Input: part model. Units: mm. Frame: model coordinates. A direction names the side the tool comes from. Round coordinates to 2 decimals unless told otherwise and drop trailing zeros. Loops run counter-clockwise (first coordinate to the right, second up) from the corner with the lowest first, then second, coordinate; pieces in that order, holes last. Notation, with made-up numbers: M 32.5,-39.5 L 39.5,-39.5 A33 cw 39.5,-0.5 Z; hole C 78,57 d3. An arc over 180 degrees is marked long. Return JSON: item names as keys, results as strings. Group by question number.
1) Material intervals for line 1 (Y direction, x = 4, z = 0.5); line 2 (Z direction, x = -3.5, y = 0); line 3 (Y direction, x = 1, z = 2.75), sorted ascending. Write a range as from..to.
2) Section B-B (z = -1.5). Output: boundary loops of the cut face in (x, y), plus the area to 3 significant figures.
3) Contact query for flat-ended pins moving along their axis: P1, Ø1.5, axis at y = -0.5, z = 0.5, coming from the +X side; P2, Ø3.5, axis at x = 0.5, y = 3, coming from the -Z side; P3, Ø0.7, axis at y = -6.5, z = 1, coming from the -X side. Output: stop coordinate, or through.
4) Section C-C (y = 2.75). Output: boundary loops of the cut face in (x, z).
5) Section A-A (x = -11). Output: boundary loops of the cut face in (y, z).
6) Mould query, pull axis X, two halves, no side actions, for faces 1 (the face through (-16.68, -0.02, 0.59)), 2 (the face through (6, -5.817, 1)), 3 (the face through (0, 0, 0)). Classes: +X half, -X half, draft (parallel to the pull), parting line (faces both ways), or undercut.
7) Access query for faces 4 (the face through (0, 0, 1.2)), 5 (the face through (-17.164, -5.753, 0.592)), 6 (the face through (13.42, 1.36, 0.59)). Directions: +Z, -Z, +X, -X, +Y, -Y. A direction counts if a zero-diameter tool reaches every point of the face in a straight line with its end or side. Return the directions, or none.
from build123d import *

# Parameters (mm, degrees)
EXTRUDE_1_DEPTH     = 1.2
CUT_EXTRUDE_START   = -1.2
CUT_EXTRUDE_1_DEPTH = 1.2
SKETCH_3_R          = 0.6
EXTRUDE_2_DEPTH     = 0.3
SKETCH_4_W          = 31.58406245
SKETCH_4_H          = 7.800680058
EXTRUDE_3_DEPTH     = 0.6


# Read off the part's stored shape, not the designer's step: Вырез-Вытянуть-Тонкостенный1
with BuildPart() as part:
    # Эскиз1 → Бобышка-Вытянуть1 (new body)
    with BuildSketch(Plane.XY):
        with BuildLine():
            Line((-18.4888994, -6.081212357), (-16.002013835, -6.217213911))
            Line((-16.002013835, -6.217213911), (10.732005982, -6.217213911))
            add(Edge.make_bspline(
                [(10.732005982, -6.217213911), (11.47341135, -6.18385268), (12.922426791, -6.118650915), (15.00936311, -5.600631561), (16.935457079, -4.747576966), (18.044624718, -3.914711141), (18.600667338, -3.497182825)],
                knots=[0, 0, 0, 0, 0.261630689, 0.511335532, 0.755025064, 1, 1, 1, 1], degree=3))
            Line((18.600667338, -3.497182825), (18.870975113, -3.202301616))
            Line((18.870975113, -3.202301616), (8.829771562, 6.217213911))
            Line((8.829771562, 6.217213911), (-15.234306629, 6.217213911))
            Line((-15.234306629, 6.217213911), (-18.870975113, -5.962739267))
            Line((-18.870975113, -5.962739267), (-18.4888994, -6.081212357))
        make_face()
    extrude(amount=EXTRUDE_1_DEPTH)

    # Вырез-Вытянуть-Тонкостенный1 outline → Вырез-Вытянуть-Тонкостенный1 (cut)
    with BuildSketch(Plane.XY.offset(1.2).offset(CUT_EXTRUDE_START)):
        with BuildLine():
            Line((-16.002013835, -6.217213911), (10.732005982, -6.217213911))
            add(Edge.make_bspline(
                [(10.732005982, -6.217213911), (11.47341135, -6.18385268), (12.922426791, -6.118650915), (15.00936311, -5.600631561), (16.935457079, -4.747576966), (18.044624718, -3.914711141), (18.600667338, -3.497182825)],
                knots=[0, 0, 0, 0, 0.261630689, 0.511335532, 0.755025064, 1, 1, 1, 1], degree=3))
            Line((18.600667338, -3.497182825), (18.870975113, -3.202301616))
            Line((18.870975113, -3.202301616), (8.829771562, 6.217213911))
            Line((8.829771562, 6.217213911), (-15.234306629, 6.217213911))
            Line((-15.234306629, 6.217213911), (-18.870975113, -5.962739267))
            Line((-18.870975113, -5.962739267), (-18.4888994, -6.081212357))
            Line((-18.4888994, -6.081212357), (-16.002013835, -6.217213911))
        make_face()
        with BuildLine():
            add(Edge.make_bspline(
                [(10.723010965, -5.817213911), (11.406644912, -5.786451106), (12.090314496, -5.756131603), (13.447652329, -5.571081257), (14.109804636, -5.413655126), (15.071741231, -5.094978106), (15.387815329, -4.97510238), (16.009307585, -4.703532881), (16.315751157, -4.551234574), (17.2086095, -4.040085881), (17.756993168, -3.630363934), (18.304501391, -3.219353606)],
                knots=[0, 0, 0, 0, 0.25, 0.25, 0.5, 0.5, 0.625, 0.625, 0.75, 0.75, 1, 1, 1, 1], degree=3))
            Line((10.723010965, -5.817213911), (-15.991084501, -5.817213911))
            Line((-15.991084501, -5.817213911), (-18.37121133, -5.687050725))
            Line((-18.37121133, -5.687050725), (-14.936288713, 5.817213911))
            Line((-14.936288713, 5.817213911), (8.671520418, 5.817213911))
            Line((8.671520418, 5.817213911), (18.304501391, -3.219353606))
        make_face(mode=Mode.SUBTRACT)
    extrude(amount=CUT_EXTRUDE_1_DEPTH, mode=Mode.SUBTRACT)

    # Эскиз3 → Бобышка-Вытянуть2 (add)
    with BuildSketch(Plane.XZ.offset(5.817213911)):
        with Locations(Location((-15.391084501, 0.6, 0), (0, 0, 270))):
            Circle(SKETCH_3_R)
        with Locations(Location((-6.891084501, 0.6, 0), (0, 0, 270))):
            Circle(SKETCH_3_R)
        with Locations(Location((1.608915499, 0.6, 0), (0, 0, 270))):
            Circle(SKETCH_3_R)
        with Locations(Location((10.108915499, 0.6, 0), (0, 0, 270))):
            Circle(SKETCH_3_R)
    extrude(amount=EXTRUDE_2_DEPTH)

    # Эскиз4 → Бобышка-Вытянуть3 (add)
    with BuildSketch(Plane.XZ.offset(6.117213911)):
        with Locations((-1.579371694, 0.79934669)):
            Rectangle(SKETCH_4_W, SKETCH_4_H)
    extrude(amount=EXTRUDE_3_DEPTH)


solid = part.part
Returned:
{
 "1": {"line 1": "y = -6.72..-6.12, -5.82..5.82", "line 2": "z = 0..1.2", "line 3": "y = -6.72..-6.12"},
 "2": {"outline": "M -17.37,-6.72 L 14.21,-6.72 L 14.21,-6.12 L -17.37,-6.12 Z", "area": "19.0 mm^2"},
 "3": {"P1": "stops at x = 16.21", "P2": "stops at z = 0", "P3": "stops at x = -17.37"},
 "4": {"outline": "M -15.85,0 L 11.94,0 L 11.94,1.2 L -15.85,1.2 Z"},
 "5": {"outline": "M -6.72,-3.1 L -6.12,-3.1 L -6.12,4.7 L -6.72,4.7 Z; M -5.82,0 L 5.82,0 L 5.82,1.2 L -5.82,1.2 Z"},
 "6": {"face 1": "-X half", "face 2": "undercut", "face 3": "draft"},
 "7": {"face 4": "+Z, +X, -X, +Y", "face 5": "+Z, -Z, -X", "face 6": "+Z, -Z, +X, +Y"}
}
